Can you work these out from the model? Positions are in its coordinate system, mm. A direction names the side the tool comes from. Round coordinates to 2 decimals unless told otherwise and drop trailing zeros. Order: outer loops, then holes, each group sorted by start corner. A loop starts at its lowest first (then second) coordinate and runs counter-clockwise, first axis right, second up. Notation, with made-up numbers: M -39.5,28 L -8.5,28 A14 cw -8.5,52 Z; hole C 60.25,-16.5 d6. An arc over 180 degrees is marked long. Answer as CSV lines item,"result". Start each with the question number.
from build123d import *

# Parameters (mm, degrees)
F0_R      = 58.801
F1_DEPTH  = 6.35
F3_R      = 56.769
F4_DEPTH  = 2.794
F5_R      = 54.6989
F6_DEPTH  = 14.0716
F7_SIZE   = 5.08
F9_DEPTH  = 38.989
F10_R     = 16.51
F11_DEPTH = 46.5455
F12_W     = 25.4
F12_H     = 80.01
F13_DEPTH = 12.7


# Not quite as in the source:
# - a length typed as a fraction of an inch, garbled in the dataset ("3 / 203.2 mm" for 3/8 in), is restored


with BuildPart() as f1:
    # F0 (on Top) → F1 (new body)
    with BuildSketch(Plane.XY):
        with Locations((-105.3465, 0)):
            Circle(F0_R)
    extrude(amount=F1_DEPTH)

    # F3 (on face) → F4 (join)
    with BuildSketch(Plane.XY.offset(6.35)):
        with Locations((-105.3465, 0)):
            Circle(F3_R)
    extrude(amount=F4_DEPTH)

    # F5 (on face) → F6 (join)
    with BuildSketch(Plane.XY.offset(9.144)):
        with Locations((-105.3465, 0)):
            Circle(F5_R)
    extrude(amount=F6_DEPTH)

    # F7
    f7_edges = [f1.edges().sort_by_distance(p)[0] for p in [
        (-160.0454, 0, 23.2156),
    ]]
    chamfer(f7_edges, length=F7_SIZE)

    # F8 (on offset) → F9 (join)
    with BuildSketch(Plane.XZ.offset(19.431)):
        Polygon((-139.2555, 9.271), (-46.5455, 9.271), (-46.5455, 70.231), (-139.2555, 23.241), align=None)
    extrude(amount=-F9_DEPTH)

    # F10 (on Right) → F11 (join, through all)
    with BuildSketch(Plane.YZ):
        with Locations((0, 50.8)):
            Circle(F10_R)
    extrude(amount=-F11_DEPTH)

    # F12 (on Front) → F13 (join, symmetric)
    with BuildSketch(Plane.XZ):
        with Locations((-93.5355, 63.2206)):
            Rectangle(F12_W, F12_H)
    extrude(amount=F13_DEPTH, both=True)

    # F14: F1 across plane


with BuildPart() as f1_1:
    add(f1.part)
    add(f1.part.mirror(Plane.YZ))


solid = f1_1.part
(1) If we mould it in two halves opening along Z, with no side actions, what happens to faces 1 (the flat face through (48, 0, 9.271)), 2 (the flat face through (-106.236, 0, 71)), 3 (the flat face through (94, 0, 103.226))? For each: +Z half, -Z half, draft (parallel to the pull), parting line (faces both ways), or undercut.
(2) If I drill on line 1 along X through (y, z) = (-12, 58); line 2 along Y through (x, z) = (112, 25.5); line 3 along Z through (x, y) = (77.5, 27.5), over which ranges is the centre line in solid material (lowest first)?
(3) I want a section at A-A on z = 15. Write out the boundary of the cut face in (x, y), and give its area (3 significant figures).
(4) I'm going to push flat-ended pins straight in: P1, Ø7.5, axis at x = -99.5, z = 80.5, coming from the +Y side; P2, Ø1, axis at x = -105, z = 51, coming from the -Y side; P3, Ø6, axis at x = -86, z = 40, coming from the +Y side; P4, Ø8, axis at x = 5, z = 29, coming from the +Y side (3 decimals). Where does each tip first touch, or does it pass through?
(5) I want a section at B-B on z = 85.5. Write out the boundary of the cut face in (x, y), and give its area (3 significant figures).
(6) For faces 4 (the flat face through (108, -21, 23.216)), 5 (the flat face through (106.236, 0, 71)), 6 (the flat face through (94, -12.7, 72)), 7 (the flat face through (94, 12.7, 72)), which set-ups out of +Z, -Z, +X, -X, +Y, -Y let a thin tool reach every point of the face, with its end or its side?
From the geometry:
1,face 1,"undercut"
1,face 2,"draft"
1,face 3,"+Z half"
2,line 1,"-106.24 to -80.84, -70.68 to 70.68, 80.84 to 106.24"
2,line 2,"-19.43 to 19.56"
2,line 3,"0 to 23.22"
3,outline,"M -54.26,19.56 A54.7 ccw long -54.22,-19.43 L -46.55,-19.43 L -46.55,19.56 Z; M 46.55,-19.43 L 54.22,-19.43 A54.7 ccw long 54.26,19.56 L 46.55,19.56 Z"
3,area,"19,200 mm²"
4,P1,"y = 12.7"
4,P2,"y = -12.7"
4,P3,"y = 19.56"
4,P4,"through"
5,outline,"M -106.24,-12.7 L -80.84,-12.7 L -80.84,12.7 L -106.24,12.7 Z; M 80.84,-12.7 L 106.24,-12.7 L 106.24,12.7 L 80.84,12.7 Z"
5,area,"1,290 mm²"
6,face 4,"+Z, +X"
6,face 5,"+Z, +X, +Y, -Y"
6,face 6,"+Z, +X, -Y"
6,face 7,"+Z, +X, +Y"
